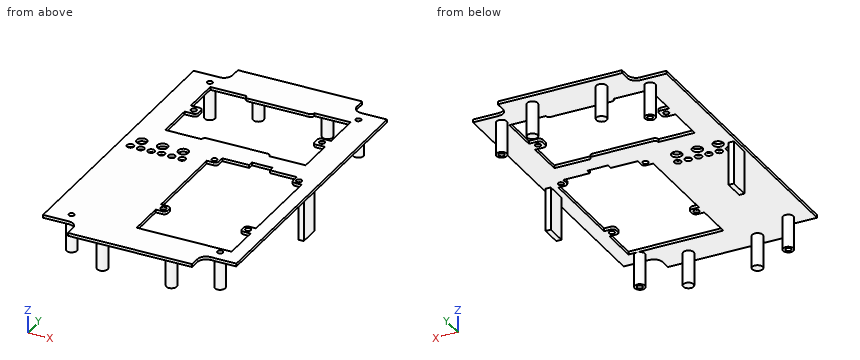
from build123d import *

# Parameters (mm, degrees)
F0_R     = 1.6
F0_R_2   = 2
F0_R_3   = 3
F2_DEPTH = 1.7
F3_R     = 1.6
F4_DEPTH = 1.701
F5_R     = 3
F5_R_2   = 1.6
F6_DEPTH = 19
F1_R     = 1.5875
F7_DEPTH = 20.701
F5_W     = 3
F5_H     = 12
F8_DEPTH = 25


# Not quite as in the source:
# - a feature names something its author has since deleted; it is built from what else it names


with BuildPart() as f2:
    # F0 (on Top) → F2 (new body)
    with BuildSketch(Plane.XY):
        with BuildLine():
            Line((36, 90), (36, 96))
            Line((36, 96), (-36, 96))
            Line((-36, 96), (-36, 90))
            ThreePointArc((-36, 90), (-37.4644660941, 86.4644660941), (-41, 85))
            Line((-41, 85), (-56, 85))
            Line((-56, 85), (-56, -85))
            Line((-56, -85), (-41, -85))
            ThreePointArc((-41, -85), (-37.4644660941, -86.4644660941), (-36, -90))
            Line((-36, -90), (-36, -96))
            Line((-36, -96), (36, -96))
            Line((36, -96), (36, -90))
            ThreePointArc((36, -90), (37.4644660941, -86.4644660941), (41, -85))
            Line((41, -85), (56, -85))
            Line((56, -85), (56, 85))
            Line((56, 85), (41, 85))
            ThreePointArc((41, 85), (37.4644660941, 86.4644660941), (36, 90))
        make_face()
        with Locations((-43, -78)):
            Circle(F0_R, mode=Mode.SUBTRACT)
        with Locations((43, -78)):
            Circle(F0_R, mode=Mode.SUBTRACT)
        with Locations((-49, 0)):
            Circle(F0_R_2, mode=Mode.SUBTRACT)
        with Locations((-43, 0)):
            Circle(F0_R_2, mode=Mode.SUBTRACT)
        with Locations((-46, 7.1000065655)):
            Circle(F0_R_3, mode=Mode.SUBTRACT)
        with Locations((-37, 0)):
            Circle(F0_R_2, mode=Mode.SUBTRACT)
        with Locations((-31, 0)):
            Circle(F0_R_2, mode=Mode.SUBTRACT)
        with Locations((-34, 7.0999998483)):
            Circle(F0_R_3, mode=Mode.SUBTRACT)
        with Locations((-25, 0)):
            Circle(F0_R_2, mode=Mode.SUBTRACT)
        with Locations((-22, 7.0999931312)):
            Circle(F0_R_3, mode=Mode.SUBTRACT)
        with Locations((-19, 0)):
            Circle(F0_R_2, mode=Mode.SUBTRACT)
        with Locations((-43, 78)):
            Circle(F0_R, mode=Mode.SUBTRACT)
        with Locations((43, 78)):
            Circle(F0_R, mode=Mode.SUBTRACT)
    extrude(amount=-F2_DEPTH)

    # F3 (on face) → F4 (cut, through all)
    with BuildSketch(Plane.XY):
        with BuildLine():
            Line((-6.8923553079, -74.973076582), (48.1076446921, -74.973076582))
            Line((48.1076446921, -74.973076582), (48.1076446921, -53.5361680277))
            Line((48.1076446921, -53.5361680277), (44.1514502317, -53.5361680277))
            ThreePointArc((44.1514502317, -53.5361680277), (42.7372366693, -52.95038159), (42.1514502317, -51.5361680277))
            Line((42.1514502317, -51.5361680277), (42.1514502317, -49.5361680277))
            ThreePointArc((42.1514502317, -49.5361680277), (42.7372366693, -48.1219544653), (44.1514502317, -47.5361680277))
            Line((44.1514502317, -47.5361680277), (48.1076446921, -47.5361680277))
            Line((48.1076446921, -47.5361680277), (48.1076446921, 4.0900148638))
            Line((48.1076446921, 4.0900148638), (44.1514502317, 4.0900148638))
            ThreePointArc((44.1514502317, 4.0900148638), (42.7372366693, 4.6758013014), (42.1514502317, 6.0900148638))
            Line((42.1514502317, 6.0900148638), (42.1514502317, 10.026923418))
            Line((42.1514502317, 10.026923418), (26.6076446921, 10.026923418))
            Line((26.6076446921, 10.026923418), (26.6076446921, 13.026923418))
            Line((26.6076446921, 13.026923418), (14.6076446921, 13.026923418))
            Line((14.6076446921, 13.026923418), (14.6076446921, 10.026923418))
            Line((14.6076446921, 10.026923418), (-0.9361608475, 10.026923418))
            Line((-0.9361608475, 10.026923418), (-0.9361608475, 6.0900148638))
            ThreePointArc((-0.9361608475, 6.0900148638), (-1.5219472852, 4.6758013014), (-2.9361608475, 4.0900148638))
            Line((-2.9361608475, 4.0900148638), (-6.8923553079, 4.0900148638))
            Line((-6.8923553079, 4.0900148638), (-6.8923553079, -47.5361680277))
            Line((-6.8923553079, -47.5361680277), (-2.9361608475, -47.5361680277))
            ThreePointArc((-2.9361608475, -47.5361680277), (-1.5219472852, -48.1219544653), (-0.9361608475, -49.5361680277))
            Line((-0.9361608475, -49.5361680277), (-0.9361608475, -51.5361680277))
            ThreePointArc((-0.9361608475, -51.5361680277), (-1.5219472852, -52.95038159), (-2.9361608475, -53.5361680277))
            Line((-2.9361608475, -53.5361680277), (-6.8923553079, -53.5361680277))
            Line((-6.8923553079, -53.5361680277), (-6.8923553079, -74.973076582))
        make_face()
        with Locations((-3.8923553079, -50.473076582)):
            Circle(F3_R)
        with Locations((45.1076446921, -50.473076582)):
            Circle(F3_R)
        with Locations((-3.8923553079, 7.026923418)):
            Circle(F3_R)
        with Locations((45.1076446921, 7.026923418)):
            Circle(F3_R)
    extrude(amount=-F4_DEPTH, mode=Mode.SUBTRACT)

    # F5 (on face) → F6 (join)
    with BuildSketch(Plane(origin=(0, 0, -1.7), x_dir=(1, 0, 0), z_dir=(0, 0, -1))):
        with Locations((-20, 88)):
            Circle(F5_R)
        with Locations((20, 88)):
            Circle(F5_R)
        with Locations((-20, -88)):
            Circle(F5_R)
        with Locations((20, -88)):
            Circle(F5_R)
        with Locations((-43, 78)):
            Circle(F5_R)
        with Locations((-43, 78)):
            Circle(F5_R_2, mode=Mode.SUBTRACT)
        with Locations((43, 78)):
            Circle(F5_R)
        with Locations((43, 78)):
            Circle(F5_R_2, mode=Mode.SUBTRACT)
        with Locations((43, -78)):
            Circle(F5_R)
        with Locations((43, -78)):
            Circle(F5_R_2, mode=Mode.SUBTRACT)
        with Locations((-43, -78)):
            Circle(F5_R)
        with Locations((-43, -78)):
            Circle(F5_R_2, mode=Mode.SUBTRACT)
    extrude(amount=F6_DEPTH)

    # F1 (on face) → F7 (cut, through all)
    with BuildSketch(Plane.XY):
        with BuildLine():
            Line((-40.6379473025, 44.8732740056), (-40.6379473025, 23.0366364121))
            Line((-40.6379473025, 23.0366364121), (-19.6368917197, 23.0366364121))
            ThreePointArc((-19.6368917197, 23.0366364121), (-19.0511052821, 24.4508499745), (-17.6368917197, 25.0366364121))
            Line((-17.6368917197, 25.0366364121), (17.6409971148, 25.0366364121))
            ThreePointArc((17.6409971148, 25.0366364121), (19.0552106772, 24.4508499745), (19.6409971148, 23.0366364121))
            Line((19.6409971148, 23.0366364121), (40.6420526975, 23.0366364121))
            Line((40.6420526975, 23.0366364121), (40.6420526975, 44.8732740056))
            Line((40.6420526975, 44.8732740056), (35.6420526975, 44.8732740056))
            ThreePointArc((35.6420526975, 44.8732740056), (34.2278391352, 45.4590604432), (33.6420526975, 46.8732740056))
            Line((33.6420526975, 46.8732740056), (33.6420526975, 49.8732740056))
            ThreePointArc((33.6420526975, 49.8732740056), (34.2278391352, 51.287487568), (35.6420526975, 51.8732740056))
            Line((35.6420526975, 51.8732740056), (40.6420526975, 51.8732740056))
            Line((40.6420526975, 51.8732740056), (40.6420526975, 73.8366364121))
            Line((40.6420526975, 73.8366364121), (19.6409971148, 73.8366364121))
            ThreePointArc((19.6409971148, 73.8366364121), (19.0552106772, 72.4224228498), (17.6409971148, 71.8366364121))
            Line((17.6409971148, 71.8366364121), (-17.6368917197, 71.8366364121))
            ThreePointArc((-17.6368917197, 71.8366364121), (-19.0511052821, 72.4224228498), (-19.6368917197, 73.8366364121))
            Line((-19.6368917197, 73.8366364121), (-40.6379473025, 73.8366364121))
            Line((-40.6379473025, 73.8366364121), (-40.6379473025, 51.8732740056))
            Line((-40.6379473025, 51.8732740056), (-35.6379473025, 51.8732740056))
            ThreePointArc((-35.6379473025, 51.8732740056), (-34.2237337401, 51.287487568), (-33.6379473025, 49.8732740056))
            Line((-33.6379473025, 49.8732740056), (-33.6379473025, 46.8732740056))
            ThreePointArc((-33.6379473025, 46.8732740056), (-34.2237337401, 45.4590604432), (-35.6379473025, 44.8732740056))
            Line((-35.6379473025, 44.8732740056), (-40.6379473025, 44.8732740056))
        make_face()
        with Locations((-37.1379473025, 48.3732740056)):
            Circle(F1_R)
        with Locations((37.1379473025, 48.3732740056)):
            Circle(F1_R)
    extrude(amount=-F7_DEPTH, mode=Mode.SUBTRACT)

    # F5 (on face) → F8 (join)
    with BuildSketch(Plane(origin=(0, 0, -1.7), x_dir=(1, 0, 0), z_dir=(0, 0, -1))):
        with Locations((53, 0)):
            Rectangle(F5_W, F5_H)
        with Locations((-53, 0)):
            Rectangle(F5_W, F5_H)
    extrude(amount=F8_DEPTH)


solid = f2.part
The listing builds one solid part. Answer for the finished solid, in the listing's coordinates (mm). Coordinates: 2 decimals unless noted, no trailing zeros. Order: outer loops, then holes, each group sorted by start corner. A loop starts at its lowest first (then second) coordinate and runs counter-clockwise, first axis right, second up.
Q1. Given P1, Ø6, axis at x = 39, z = -18.5, coming from the +Y side; P2, Ø1.8, axis at x = -43, y = -78, coming from the -Z side; P3, Ø10, axis at x = -3.5, y = 7, coming from the -Z side; P4, Ø3.5, axis at x = -43, y = -78, coming from the -Z side, each flat-ended and moving along its own axis, determine where each tip first touches the part or whether it passes through.
Q2. A cutting plane is placed at D-D, the plane x = 7.5. Write down the section's boundary in (y, z).
Q3. Consider line 1 (Y direction, x = -43, z = -14.5); line 2 (X direction, y = -78, z = -0.35); line 3 (X direction, y = 87.5, z = -17.25). Determine where each line is inside the solid, lowest interval first.
Q4. A cutting plane is placed at C-C, the plane x = -9. Write down the section's boundary in (y, z), and give its area (3 significant figures).
Q5. A cutting plane is placed at A-A, the plane z = -15. State how many separate pieces and enclosed holes the cut face has, and give its area (3 significant figures).
Q6. A cutting plane is placed at B-B, the plane y = 59. Write down the section's boundary in (x, z).
Answers follow:
1. P1: stops at y = 80.83
1. P2: passes through
1. P3: stops at z = -1.7
1. P4: stops at z = -20.7
2. outline: (-96, -1.7) - (-74.97, -1.7) - (-74.97, 0) - (-96, 0) - close; (10.03, -1.7) - (25.04, -1.7) - (25.04, 0) - (10.03, 0) - close; (71.84, -1.7) - (96, -1.7) - (96, 0) - (71.84, 0) - close
3. line 1: y = -81 to -79.6, -76.4 to -75, 75 to 76.4, 79.6 to 81
3. line 2: x = -56 to -44.6, -41.4 to 41.4, 44.6 to 56
3. line 3: x = -22.96 to -17.04, 17.04 to 22.96
4. outline: (-96, -1.7) - (25.04, -1.7) - (25.04, 0) - (-96, 0) - close; (71.84, -1.7) - (96, -1.7) - (96, 0) - (71.84, 0) - close
4. area: 247 mm2
5. separate pieces: 10
5. enclosed holes: 4
5. area: 266 mm2
6. outline: (-56, -1.7) - (-40.64, -1.7) - (-40.64, 0) - (-56, 0) - close; (40.64, -1.7) - (56, -1.7) - (56, 0) - (40.64, 0) - close
